Verification items for the finished model (mm, model axes). Face numbers are marked on the shaded views. A direction names the side the tool comes from. Coordinates: 2 decimals unless noted, no trailing zeros. Write each loop counter-clockwise with the first axis right and the second up, starting at its lowest first coordinate (ties: lowest second). Pieces come first, ordered by that corner, then holes. Notation, with made-up numbers: (-2.5, 0) -> (49.5, 0) arc R14 ccw to (49.5, 17) -> close; hole circle Ø11 at (52, -7.5). An arc over 180 degrees is marked (long way). Answer in a Markdown table with one row per item.
```python
from build123d import *

# Parameters (mm, degrees)
BOSS_EXTRUDE1_DEPTH  = 2.5
M8_CLEARANCE_HOLE1_D = 9.25
SKETCH4_R            = 4.937986177
BOSS_EXTRUDE2_DEPTH  = 1.3
SKETCH5_R            = 5.099596851
BOSS_EXTRUDE3_DEPTH  = 3
CUT_EXTRUDE1_DEPTH   = 3.6
FILLET1_R            = 1.5
SKETCH11_R           = 2.5
CUT_EXTRUDE2_DEPTH   = 10


with BuildPart() as part:
    # Sketch1 → Boss-Extrude1 (new body)
    with BuildSketch(Plane.XY.offset(2.5)):
        with BuildLine():
            Line((4, -8.419183588), (4, -4))
            Line((4, -4), (8.419183588, -4))
            Line((8.419183588, -4), (17.898853189, -2.467978147))
            ThreePointArc((17.898853189, -2.467978147), (20, 0), (17.898853189, 2.467978147))
            Line((17.898853189, 2.467978147), (8.419183588, 4))
            Line((8.419183588, 4), (4, 4))
            Line((4, 4), (4, 8.419183588))
            Line((4, 8.419183588), (2.467978147, 17.898853189))
            ThreePointArc((2.467978147, 17.898853189), (0, 20), (-2.467978147, 17.898853189))
            Line((-2.467978147, 17.898853189), (-4, 8.419183588))
            Line((-4, 8.419183588), (-4, 4))
            Line((-4, 4), (-8.419183588, 4))
            Line((-8.419183588, 4), (-17.898853189, 2.467978147))
            ThreePointArc((-17.898853189, 2.467978147), (-20, 0), (-17.898853189, -2.467978147))
            Line((-17.898853189, -2.467978147), (-8.419183588, -4))
            Line((-8.419183588, -4), (-4, -4))
            Line((-4, -4), (-4, -8.419183588))
            Line((-4, -8.419183588), (-2.467978147, -17.898853189))
            ThreePointArc((-2.467978147, -17.898853189), (0, -20), (2.467978147, -17.898853189))
            Line((2.467978147, -17.898853189), (4, -8.419183588))
        make_face()
    extrude(amount=-BOSS_EXTRUDE1_DEPTH)

    # M8 Clearance Hole1 (through all)
    with Locations(Plane.XY.offset(2.5)):
        with Locations((0, 0)):
            Hole(M8_CLEARANCE_HOLE1_D / 2)

    # Sketch4 → Boss-Extrude2 (add)
    with BuildSketch(Plane(origin=(0, 0, 2), x_dir=(-1, 0, 0), z_dir=(0, 0, -1))):
        with Locations(Location((0, 0, 0), (0, 0, 180))):
            Circle(SKETCH4_R)
    extrude(amount=-BOSS_EXTRUDE2_DEPTH)

    # Sketch5 → Boss-Extrude3 (add)
    with BuildSketch(Plane.XY):
        with Locations(Location((0, 0, 0), (0, 0, 180))):
            Circle(SKETCH5_R)
    extrude(amount=-BOSS_EXTRUDE3_DEPTH)

    # Sketch6 → Cut-Extrude1 (cut)
    with BuildSketch(Plane(origin=(0, 0, -3), x_dir=(-1, 0, 0), z_dir=(0, 0, -1))):
        with BuildLine():
            Line((-2.994554723, 0.180671), (-2.667483, 0))
            Line((-2.667483, 0), (-2.993563417, -0.196413))
            ThreePointArc((-2.993563417, -0.196413), (-2.975345367, -0.383822804), (-2.94540633, -0.569720588))
            Line((-2.94540633, -0.569720588), (-2.583679116, -0.663376046))
            Line((-2.583679116, -0.663376046), (-2.850669191, -0.934711273))
            ThreePointArc((-2.850669191, -0.934711273), (-2.786416572, -1.111702609), (-2.711187226, -1.284314536))
            Line((-2.711187226, -1.284314536), (-2.337533172, -1.285069736))
            Line((-2.337533172, -1.285069736), (-2.528656935, -1.614278199))
            ThreePointArc((-2.528656935, -1.614278199), (-2.422406975, -1.76973005), (-2.306614256, -1.918210278))
            Line((-2.306614256, -1.918210278), (-1.944511421, -1.826017768))
            Line((-1.944511421, -1.826017768), (-2.047759865, -2.192414089))
            ThreePointArc((-2.047759865, -2.192414089), (-1.906188639, -2.316558843), (-1.75710823, -2.431577814))
            Line((-1.75710823, -2.431577814), (-1.429308867, -2.252230388))
            Line((-1.429308867, -2.252230388), (-1.438194511, -2.632792538))
            ThreePointArc((-1.438194511, -2.632792538), (-1.27019746, -2.717829725), (-1.097196632, -2.792160373))
            Line((-1.097196632, -2.792160373), (-0.824297579, -2.536927089))
            Line((-0.824297579, -2.536927089), (-0.738262106, -2.90774295))
            ThreePointArc((-0.738262106, -2.90774295), (-0.554395104, -2.948329369), (-0.368344134, -2.977301227))
            Line((-0.368344134, -2.977301227), (-0.167492643, -2.662219332))
            Line((-0.167492643, -2.662219332), (0.008058022, -2.999989178))
            ThreePointArc((0.008058022, -2.999989178), (0.196241936, -2.993574636), (0.383652781, -2.975367296))
            Line((0.383652781, -2.975367296), (0.499836471, -2.620234542))
            Line((0.499836471, -2.620234542), (0.753871834, -2.903735053))
            ThreePointArc((0.753871834, -2.903735053), (0.934548373, -2.850722599), (1.11154338, -2.786480094))
            Line((1.11154338, -2.786480094), (1.135759022, -2.41361078))
            Line((1.135759022, -2.41361078), (1.452317107, -2.625028575))
            ThreePointArc((1.452317107, -2.625028575), (1.614133699, -2.528749177), (1.769591621, -2.4225081))
            Line((1.769591621, -2.4225081), (1.700317656, -2.055330976))
            Line((1.700317656, -2.055330976), (2.059507955, -2.181381898))
            ThreePointArc((2.059507955, -2.181381898), (2.192297068, -2.047885144), (2.316449912, -1.906321013))
            Line((2.316449912, -1.906321013), (2.158039079, -1.567907168))
            Line((2.158039079, -1.567907168), (2.537292343, -1.600670974))
            ThreePointArc((2.537292343, -1.600670974), (2.63271035, -1.438344956), (2.717757136, -1.270352765))
            Line((2.717757136, -1.270352765), (2.48016297, -0.981965986))
            Line((2.48016297, -0.981965986), (2.855649322, -0.919384005))
            ThreePointArc((2.855649322, -0.919384005), (2.907700758, -0.738428265), (2.948297684, -0.554563582))
            Line((2.948297684, -0.554563582), (2.6464491, -0.33432427))
            Line((2.6464491, -0.33432427), (2.994575352, -0.180328758))
            ThreePointArc((2.994575352, -0.180328758), (2.999989634, 0.007886591), (2.993585845, 0.196070871))
            Line((2.993585845, 0.196070871), (2.6464491, 0.33432427))
            Line((2.6464491, 0.33432427), (2.945341199, 0.570057208))
            ThreePointArc((2.945341199, 0.570057208), (2.903778127, 0.753705902), (2.850775998, 0.93438547))
            Line((2.850775998, 0.93438547), (2.48016297, 0.981965986))
            Line((2.48016297, 0.981965986), (2.711040427, 1.284624383))
            ThreePointArc((2.711040427, 1.284624383), (2.625111562, 1.4521671), (2.528841411, 1.613989194))
            Line((2.528841411, 1.613989194), (2.158039079, 1.567907168))
            Line((2.158039079, 1.567907168), (2.306395014, 1.918473883))
            ThreePointArc((2.306395014, 1.918473883), (2.181499583, 2.059383299), (2.048010417, 2.192180041))
            Line((2.048010417, 2.192180041), (1.700317656, 2.055330976))
            Line((1.700317656, 2.055330976), (1.756830319, 2.431778614))
            ThreePointArc((1.756830319, 2.431778614), (1.600815962, 2.53720087), (1.438495397, 2.632628153))
            Line((1.438495397, 2.632628153), (1.135759022, 2.41361078))
            Line((1.135759022, 2.41361078), (1.096877515, 2.792285751))
            ThreePointArc((1.096877515, 2.792285751), (0.919547186, 2.85559678), (0.73859442, 2.907658557))
            Line((0.73859442, 2.907658557), (0.499836471, 2.620234542))
            Line((0.499836471, 2.620234542), (0.368003863, 2.977343305))
            ThreePointArc((0.368003863, 2.977343305), (0.180499879, 2.994565042), (-0.00771516, 2.999990079))
            Line((-0.00771516, 2.999990079), (-0.167492643, 2.662219332))
            Line((-0.167492643, 2.662219332), (-0.383992826, 2.975323429))
            ThreePointArc((-0.383992826, 2.975323429), (-0.569888899, 2.94537377), (-0.753539968, 2.903821192))
            Line((-0.753539968, 2.903821192), (-0.824297579, 2.536927089))
            Line((-0.824297579, 2.536927089), (-1.111861833, 2.78635304))
            ThreePointArc((-1.111861833, 2.78635304), (-1.284469462, 2.711113831), (-1.452017089, 2.62519454))
            Line((-1.452017089, 2.62519454), (-1.429308867, 2.252230388))
            Line((-1.429308867, 2.252230388), (-1.769868472, 2.422305842))
            ThreePointArc((-1.769868472, 2.422305842), (-1.918342084, 2.306504639), (-2.059258636, 2.18161726))
            Line((-2.059258636, 2.18161726), (-1.944511421, 1.826017768))
            Line((-1.944511421, 1.826017768), (-2.316667766, 1.906056259))
            ThreePointArc((-2.316667766, 1.906056259), (-2.431678218, 1.756969278), (-2.53710939, 1.600960944))
            Line((-2.53710939, 1.600960944), (-2.337533172, 1.285069736))
            Line((-2.337533172, 1.285069736), (-2.717902304, 1.270042151))
            ThreePointArc((-2.717902304, 1.270042151), (-2.792223067, 1.097037075), (-2.855544229, 0.919710365))
            Line((-2.855544229, 0.919710365), (-2.583679116, 0.663376046))
            Line((-2.583679116, 0.663376046), (-2.948361045, 0.554226624))
            ThreePointArc((-2.948361045, 0.554226624), (-2.977322271, 0.368173999), (-2.994554723, 0.180671))
        make_face()
    extrude(amount=-CUT_EXTRUDE1_DEPTH, mode=Mode.SUBTRACT)

    # Sketch9 → CBORE for M2.5 Hex Head Machine Screw1 (revolve, cut)
    with BuildSketch(Plane(origin=(0, 0, 3.3), x_dir=(0, -1, 0), z_dir=(1, 0, 0))):
        Polygon((0, 0), (0, 1.3), (1.5, 1.3), (1.5, 1.5), (2.85, 1.5), (2.85, 0), align=None)
    revolve(axis=Axis((0, 0, 9.65), (0, 0, -1)), mode=Mode.SUBTRACT)

    # Fillet1
    fillet1_edges = [part.edges().sort_by_distance(p)[0] for p in [
        (-4, -4, 1.25),
        (-4, 4, 1.25),
        (4, 4, 1.25),
        (4, -4, 1.25),
    ]]
    fillet(fillet1_edges, radius=FILLET1_R)

    # Sketch11 → Cut-Extrude2 (cut)
    with BuildSketch(Plane.XY.offset(2.5)):
        with Locations((-10, 0)):
            Circle(SKETCH11_R)
        with Locations((10, 0)):
            Circle(SKETCH11_R)
        with Locations((0, -10)):
            Circle(SKETCH11_R)
        with Locations((0, 10)):
            Circle(SKETCH11_R)
    extrude(amount=-CUT_EXTRUDE2_DEPTH, mode=Mode.SUBTRACT)


solid = part.part
```
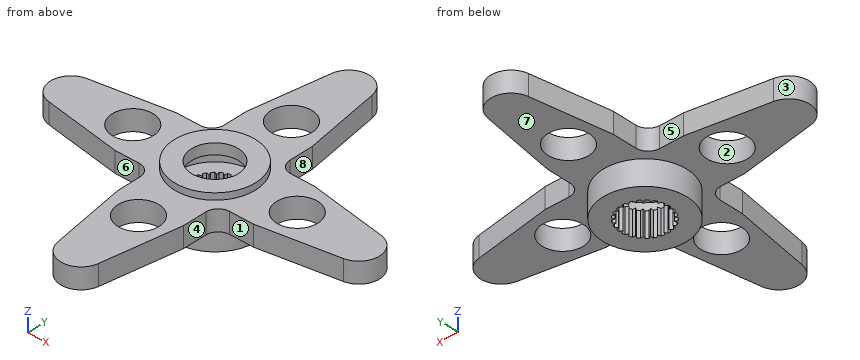
1. Depth check by flat-ended pin: P1, Ø3, axis at y = 6.5, z = 1.5, coming from the +X side; P2, Ø6.5, axis at x = 0, y = 10, coming from the +Z side; P3, Ø2, axis at x = -6, z = 2, coming from the +Y side. Enter the tip coordinate at first touch or a pass-through.
Geometry says:
| item | result |
|---|---|
| P1 | x = 4.09 |
| P2 | z = 2.5 |
| P3 | y = 4.09 |
2. Mould release check, pull along X, two halves, no side actions. Record for the marked faces 1, 2, 3 and 4: released by +X, released by -X, zero draft, split by the parting line, or undercut.
Geometry says:
| item | result |
|---|---|
| face 1 | zero draft |
| face 2 | undercut |
| face 3 | released by -X |
| face 4 | released by +X |
3. Section check D-D, the plane y = 3.5. Record the boundary of the cut face in (x, z), plus the area to 3 significant figures.
Geometry says:
| item | result |
|---|---|
| outline | (-11.51, 0) -> (-3.71, 0) -> (-3.71, -3) -> (3.71, -3) -> (3.71, 0) -> (11.51, 0) -> (11.51, 2.5) -> (3.48, 2.5) -> (3.48, 3.3) -> (-3.48, 3.3) -> (-3.48, 2.5) -> (-11.51, 2.5) -> close; hole (-3.02, 0) -> (3.02, 0) -> (3.02, 2) -> (-3.02, 2) -> close |
| area | 73.3 mm^2 |
4. Thickness scan on line 1 (Y direction, x = 0, z = 1.5) (3 decimals); line 2 (Y direction, x = 0, z = 2.8); line 3 (X direction, y = 11, z = 2). Record the ranges inside material, lowest first. Write a range as from..to.
Geometry says:
| item | result |
|---|---|
| line 1 | -20..-12.5, -7.5..-4.625, 4.625..7.5, 12.5..20 |
| line 2 | -4.94..-2.85, 2.85..4.94 |
| line 3 | -3.58..-2.29, 2.29..3.58 |
5. Section check A-A, the plane z = 1.25. State how many separate pieces and enclosed holes the cut face has, plus the area to 3 significant figures.
Geometry says:
| item | result |
|---|---|
| separate pieces | 1 |
| enclosed holes | 5 |
| area | 338 mm^2 |
6. Tool access check on the marked faces 5, 6, 7 and 8. Record the directions out of +Z, -Z, +X, -X, +Y, -Y that give a thin tool (end or side, any length) a straight path to the whole face; none if there is none.
Geometry says:
| item | result |
|---|---|
| face 5 | +Z, -Z, -X, +Y |
| face 6 | +Z, -Z, -X, -Y |
| face 7 | -Z |
| face 8 | +Z, -Z, +X, +Y |
7. Section check B-B, the plane y = -10. Record the boundary of the cut face in (x, z), plus the area to 3 significant figures.
Geometry says:
| item | result |
|---|---|
| outline | (-3.74, 0) -> (-2.5, 0) -> (-2.5, 2.5) -> (-3.74, 2.5) -> close; (2.5, 0) -> (3.74, 0) -> (3.74, 2.5) -> (2.5, 2.5) -> close |
| area | 6.22 mm^2 |
